Autodesk Fusion 360 part; units mm, degrees
sketch "Sketch1" plane through (0, 0, 0) normal (0, 0, 1) x (1, 0, 0)
  line L0 (-9, -12) -> (-9, 12)
  line L1 (9, 12) -> (9, -12)
  line L2 (9, -21) -> (-9, 21) construction
  line L3 (-9, -21) -> (9, 21) construction
  line L4 (9, -7.5) -> (-9, -7.5)
  line L5 (-9, -7.5) -> (-9, 7.5)
  line L6 (-9, 7.5) -> (9, 7.5)
  line L7 (9, 7.5) -> (9, -7.5)
  line L8 (9, -7.5) -> (-9, 7.5) construction
  line L9 (-9, -7.5) -> (9, 7.5) construction
  circle A0 centre (0, 0) radius 2.75
  arc A1 (0, 21) -> (-9, 12) centre (0, 12) ccw
  arc A2 (9, 12) -> (0, 21) centre (0, 12) ccw
  arc A3 (0, -21) -> (9, -12) centre (0, -12) ccw
  arc A4 (-9, -12) -> (0, -21) centre (0, -12) ccw
  line L10 (0, -21.9731) -> (0, 33.0269) construction
  line L11 (2.0496, 8.45) -> (4.0992, 12)
  line L12 (4.0992, 12) -> (2.0496, 15.55)
  line L13 (2.0496, 15.55) -> (-2.0496, 15.55)
  line L14 (-2.0496, 15.55) -> (-4.0992, 12)
  line L15 (-4.0992, 12) -> (-2.0496, 8.45)
  line L16 (-2.0496, 8.45) -> (2.0496, 8.45)
  line L17 (2.0496, -15.55) -> (4.0992, -12)
  line L18 (4.0992, -12) -> (2.0496, -8.45)
  line L19 (2.0496, -8.45) -> (-2.0496, -8.45)
  line L20 (-2.0496, -8.45) -> (-4.0992, -12)
  line L21 (-4.0992, -12) -> (-2.0496, -15.55)
  line L22 (-2.0496, -15.55) -> (2.0496, -15.55)
  circle A5 centre (0, 12) radius 2
  circle A6 centre (0, -12) radius 2
  line L23 (-9, 0) -> (0, 0) construction
  line L24 (-3.75, 3.5) -> (-7.25, 3.5)
  line L25 (-7.25, 3.5) -> (-7.25, -3.5)
  line L26 (-7.25, -3.5) -> (-3.75, -3.5)
  line L27 (-3.75, -3.5) -> (-3.75, 3.5)
  line L28 (-3.75, 3.5) -> (-7.25, -3.5) construction
  line L29 (-7.25, 3.5) -> (-3.75, -3.5) construction
  point P0 (0, 12)
  point P1 (0, -12)
  point P2 (-5.5, 0)
  dimension "d14" = 18
  dimension "d15" = 42
  dimension "d16" = 18
  dimension "d17" = 15
  dimension "d18" = 5.5
  dimension "d19" = 9
  dimension "d20" = 12
  dimension "d21" = 12
  dimension "d22" = 3.55
  dimension "d23" = 3.55
  dimension "d24" = 4
  dimension "d25" = 4
  dimension "d26" = 3.5
  dimension "d27" = 7
  dimension "d28" = 3.5
extrude "Extrude1" add sketch "Sketch1" against normal blind 5 contours L0 L1 L4 A3 A4 | L0 L1 L4 L5 L6 L7 | L0 L1 L6 A1 A2 | L11 L12 L13 L14 L15 L16 | L17 L18 L19 L20 L21 L22 | L24 L25 L26 L27
extrude "Extrude2" add sketch "Sketch1" along normal blind 10 contours L0 L1 L4 L5 L6 L7 | L24 L25 L26 L27
extrude "Extrude3" [suppressed]
extrude "Extrude7" add sketch "Sketch1" along normal blind 4 contours L0 L1 L4 A3 A4 | L0 L1 L6 A1 A2 | L11 L12 L13 L14 L15 L16 | L17 L18 L19 L20 L21 L22
extrude "Extrude4" cut sketch "Sketch1" against normal blind 5 from surface at 10 contours L24 L25 L26 L27
sketch "Sketch2" plane through (-3.75, 0, 0) normal (-1, 0, 0) x (0, 0, 1)
  line L0 (10, -3.5) -> (10, 3.5)
  line L1 (10, 3.5) -> (5, 3.5)
  line L2 (5, 3.5) -> (5, -3.5)
  line L3 (5, -3.5) -> (10, -3.5)
  line L4 (9.0415, 0) -> (7.0207, 3.5)
  line L5 (7.0207, 3.5) -> (2.9793, 3.5)
  line L6 (2.9793, 3.5) -> (0.9585, 0)
  line L7 (0.9585, 0) -> (2.9793, -3.5)
  line L8 (2.9793, -3.5) -> (7.0207, -3.5)
  line L9 (7.0207, -3.5) -> (9.0415, 0)
  circle A0 centre (5, 0) radius 2.1
  point P0 (5, 0)
  dimension "d38" = 3.5
  dimension "d41" = 4.2
extrude "Extrude5" cut sketch "Sketch2" along normal up to surface (3.5 mm away) contours L1 L2 L3 L4 L5 L8 L9 A0 | L2 L5 L6 L7 L8 A0 | L2 A0 | L2 A0
extrude "Extrude6" cut sketch "Sketch2" against normal blind 9 from surface at 5.25 contours L2 A0 | L2 A0
chamfer "Chamfer1" [suppressed]
chamfer "Chamfer2" distance 0.5 angle 45 2 edges at (-1.8647, 12.7232, 4) (-1.8647, -11.2768, 4)
The listing builds one solid part. Answer for the finished solid, in the listing's coordinates (mm). A direction names the side the tool comes from. Give positions to 0.01 mm unless a question says otherwise; leave off trailing zeros. Loops run counter-clockwise (first coordinate to the right, second up) from the corner with the lowest first, then second, coordinate; pieces in that order, holes last. Notation, with made-up numbers: M 6,22.5 L 50,22.5 A25 ccw 50,58.5 Z; hole C 13.25,-7 d7. An arc over 180 degrees is marked long. Answer as CSV lines item,"result".
Item 1: Given pin 1 Ø2 at (x, z) = (2, 3.5) entering from +Y; pin 2 Ø8 at (y, z) = (16.5, -3.5) entering from +X; pin 3 Ø7 at (x, y) = (3, -11.5) entering from +Z, each flat-ended and moving along its own axis, determine where each tip first touches the part or whether it passes through.
Values follow:
pin 1,"stops at y = 20.94"
pin 2,"stops at x = 8.99"
pin 3,"stops at z = 4"
Item 2: Straight lines are drawn through the part: line 1 along Y through (x, z) = (0, 0.5); line 2 along X through (y, z) = (-0.5, 7.75); line 3 along Y through (x, z) = (-4.75, 7.75). For each, find the intervals that lie inside material, in ascending order. Write a range as [from, to].
Values follow:
line 1,"y = [-21, -14], [-10, -2.75], [2.75, 10], [14, 21]"
line 2,"x = [-9, -7.25], [-3.75, -2.7], [2.7, 9]"
line 3,"y = [-7.5, -3.5], [3.5, 7.5]"
Item 3: Which of the six approach directions +Z, -Z, +X, -X, +Y, -Y give full straight-line access (tool end or side, diameter ignored) to faces 5 (the flat face through (2, -14, 4)), 6 (the flat face through (0, 7.5, 7)), 7 (the flat face through (-5.5, 1.8, 2)), 8 (the cylindrical face through (-2.996, 0.631, 7.003))?
Values follow:
face 5,"+Z, +X, -X, -Y"
face 6,"+Z, +X, -X, +Y"
face 7,"+Z"
face 8,"-X"
Item 4: The mould has two halves that part along X. Classify faces 1 (the flat face through (4, 0, 10)), 2 (the cylindrical face through (2.54, -1.05, 2.61)), 3 (the flat face through (-7.25, 0, 8)), 4 (the flat face through (9, 0, 1)): released by +X, released by -X, zero draft, split by the parting line, or undercut.
Values follow:
face 1,"zero draft"
face 2,"undercut"
face 3,"undercut"
face 4,"released by +X"
Item 5: The part is cut by section A-A (x = 0). Give the vertices of the cut face in (y, z), and give its area (3 significant figures).
Values follow:
outline,"M -21,-5 L -14,-5 L -14,3.5 L -14.5,4 L -21,4 Z; M -10,-5 L -2.75,-5 L -2.75,10 L -7.5,10 L -7.5,4 L -9.5,4 L -10,3.5 Z; M 2.75,-5 L 10,-5 L 10,3.5 L 9.5,4 L 7.5,4 L 7.5,10 L 2.75,10 Z; M 14,-5 L 21,-5 L 21,4 L 14.5,4 L 14,3.5 Z"
area,"313 mm^2"
Item 6: The part is cut by section C-C (y = 8.5). Give the vertices of the cut face in (x, z), and give its area (3 significant figures).
Values follow:
outline,"M -9,-5 L 9,-5 L 9,4 L -9,4 Z"
area,"162 mm^2"
Item 7: The part is cut by section D-D (z = 5.75). Give the vertices of the cut face in (x, y), and give its area (3 significant figures).
Values follow:
outline,"M -9,-7.5 L 9,-7.5 L 9,7.5 L -9,7.5 L -9,1.96 L -7.25,1.96 L -7.25,3.5 L -3.75,3.5 L -3.75,1.96 L -1.93,1.96 A2.75 cw long -1.93,-1.96 L -3.75,-1.96 L -3.75,-3.5 L -7.25,-3.5 L -7.25,-1.96 L -9,-1.96 Z"
area,"210 mm^2"
Item 8: The part is cut by section B-B (z = 7.75). Give the vertices of the cut face in (x, y), and give its area (3 significant figures).
Values follow:
outline,"M -9,-7.5 L 9,-7.5 L 9,7.5 L -9,7.5 Z; hole M -7.25,-3.5 L -3.75,-3.5 L -3.75,3.5 L -7.25,3.5 Z; hole C 0,0 d5.5"
area,"222 mm^2"
